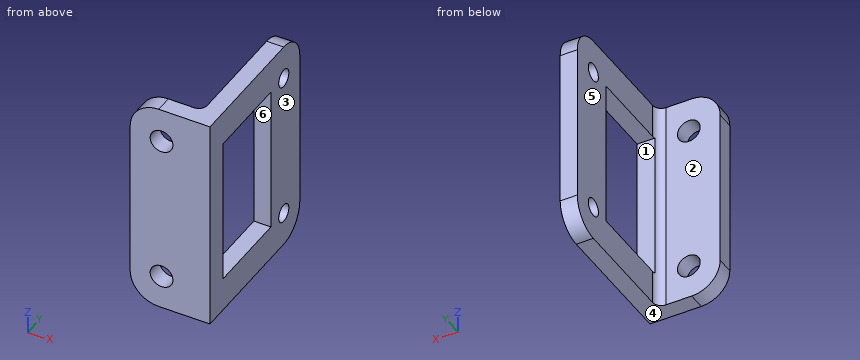
from build123d import *

# Parameters (mm, degrees)
BOSS_EXTRUDE1_DEPTH     = 19
CUT_EXTRUDE1_DEPTH      = 33.954514107
CUT_EXTRUDE1_DEPTH_BACK = 33.954514107
SKETCH2_R               = 2
SKETCH3_R               = 1.575
SKETCH3_W               = 26
SKETCH3_H               = 15
CUT_EXTRUDE2_DEPTH      = 36.580893749
FILLET1_R               = 1.5
FILLET2_R               = 5


with BuildPart() as part:
    # Sketch1 → Boss-Extrude1 (new, symmetric)
    with BuildSketch(Plane.XY):
        Polygon((0, 0), (4, 0), (4, 28), (1, 28), (1, 3), (-10, 3), (-10, 0), align=None)
    extrude(amount=BOSS_EXTRUDE1_DEPTH, both=True)

    # Sketch2 → Cut-Extrude1 (cut, two sides: drawn at the far end of the back side and taken through both)
    with BuildSketch(Plane(origin=(0, 3, 0), x_dir=(1, 0, 0), z_dir=(0, 1, 0)).offset(-CUT_EXTRUDE1_DEPTH_BACK)):
        with Locations(Location((-4.5, 13, 0), (0, 0, 180))):
            Circle(SKETCH2_R)
        with Locations((-4.5, -13)):
            Circle(SKETCH2_R)
    extrude(amount=CUT_EXTRUDE1_DEPTH + CUT_EXTRUDE1_DEPTH_BACK, mode=Mode.SUBTRACT)

    # Sketch3 → Cut-Extrude2 (cut, through all)
    with BuildSketch(Plane.ZY.offset(-1)):
        with Locations((-13, 23)):
            Circle(SKETCH3_R)
        with Locations(Location((13, 23, 0), (0, 0, 180))):
            Circle(SKETCH3_R)
        with Locations((0, 11.5)):
            Rectangle(SKETCH3_W, SKETCH3_H)
    extrude(amount=-CUT_EXTRUDE2_DEPTH, mode=Mode.SUBTRACT)

    # Fillet1
    # the kernel refuses this fillet: 1.5 mm, written as the material it adds along each edge
    with BuildSketch(Plane(origin=(1, 3, -19), x_dir=(0, 1, 0), z_dir=(0, 0, 1))) as fillet1_piece_1_section:
        with BuildLine():
            CenterArc((FILLET1_R, FILLET1_R), FILLET1_R, 180, 90)
            Line((0, FILLET1_R), (0, 0))
            Line((0, 0), (FILLET1_R, 0))
        make_face()
    fillet1_piece_1 = extrude(amount=38, mode=Mode.PRIVATE)
    fillet1_piece_1 = split(fillet1_piece_1, bisect_by=Plane(origin=(0.995303959, 4, -16), z_dir=(0, 1, 0)), keep=Keep.TOP, mode=Mode.PRIVATE)
    fillet1_piece_1 = split(fillet1_piece_1, bisect_by=Plane(origin=(0.995303959, 4.189014255, -13), z_dir=(0, 0, -1)), keep=Keep.TOP, mode=Mode.PRIVATE)
    add(fillet1_piece_1)
    with BuildSketch(Plane(origin=(1, 3, -19), x_dir=(0, 1, 0), z_dir=(0, 0, 1))) as fillet1_piece_2_section:
        with BuildLine():
            CenterArc((FILLET1_R, FILLET1_R), FILLET1_R, 180, 90)
            Line((0, FILLET1_R), (0, 0))
            Line((0, 0), (FILLET1_R, 0))
        make_face()
    fillet1_piece_2 = extrude(amount=38, mode=Mode.PRIVATE)
    fillet1_piece_2 = split(fillet1_piece_2, bisect_by=Plane(origin=(0.642494848, 4, -16), z_dir=(0, -1, 0)), keep=Keep.TOP, mode=Mode.PRIVATE)
    fillet1_piece_2 = split(fillet1_piece_2, bisect_by=Plane(origin=(0.642494848, 3.294160002, -13), z_dir=(0, 0, -1)), keep=Keep.TOP, mode=Mode.PRIVATE)
    add(fillet1_piece_2)
    with BuildSketch(Plane(origin=(1, 3, -19), x_dir=(0, 1, 0), z_dir=(0, 0, 1))) as fillet1_piece_3_section:
        with BuildLine():
            CenterArc((FILLET1_R, FILLET1_R), FILLET1_R, 180, 90)
            Line((0, FILLET1_R), (0, 0))
            Line((0, 0), (FILLET1_R, 0))
        make_face()
    fillet1_piece_3 = extrude(amount=38, mode=Mode.PRIVATE)
    fillet1_piece_3 = split(fillet1_piece_3, bisect_by=Plane(origin=(0.642494848, 4, 0), z_dir=(0, -1, 0)), keep=Keep.TOP, mode=Mode.PRIVATE)
    fillet1_piece_3 = split(fillet1_piece_3, bisect_by=Plane(origin=(0.642494848, 3.294160002, -13), z_dir=(0, 0, 1)), keep=Keep.TOP, mode=Mode.PRIVATE)
    fillet1_piece_3 = split(fillet1_piece_3, bisect_by=Plane(origin=(0.642494848, 3.294160002, 13), z_dir=(0, 0, -1)), keep=Keep.TOP, mode=Mode.PRIVATE)
    add(fillet1_piece_3)
    with BuildSketch(Plane(origin=(1, 3, -19), x_dir=(0, 1, 0), z_dir=(0, 0, 1))) as fillet1_piece_4_section:
        with BuildLine():
            CenterArc((FILLET1_R, FILLET1_R), FILLET1_R, 180, 90)
            Line((0, FILLET1_R), (0, 0))
            Line((0, 0), (FILLET1_R, 0))
        make_face()
    fillet1_piece_4 = extrude(amount=38, mode=Mode.PRIVATE)
    fillet1_piece_4 = split(fillet1_piece_4, bisect_by=Plane(origin=(0.995303959, 4, 16), z_dir=(0, 1, 0)), keep=Keep.TOP, mode=Mode.PRIVATE)
    fillet1_piece_4 = split(fillet1_piece_4, bisect_by=Plane(origin=(0.995303959, 4.189014255, 13), z_dir=(0, 0, 1)), keep=Keep.TOP, mode=Mode.PRIVATE)
    add(fillet1_piece_4)
    with BuildSketch(Plane(origin=(1, 3, -19), x_dir=(0, 1, 0), z_dir=(0, 0, 1))) as fillet1_piece_5_section:
        with BuildLine():
            CenterArc((FILLET1_R, FILLET1_R), FILLET1_R, 180, 90)
            Line((0, FILLET1_R), (0, 0))
            Line((0, 0), (FILLET1_R, 0))
        make_face()
    fillet1_piece_5 = extrude(amount=38, mode=Mode.PRIVATE)
    fillet1_piece_5 = split(fillet1_piece_5, bisect_by=Plane(origin=(0.642494848, 4, 16), z_dir=(0, -1, 0)), keep=Keep.TOP, mode=Mode.PRIVATE)
    fillet1_piece_5 = split(fillet1_piece_5, bisect_by=Plane(origin=(0.642494848, 3.294160002, 13), z_dir=(0, 0, 1)), keep=Keep.TOP, mode=Mode.PRIVATE)
    add(fillet1_piece_5)

    # Fillet2
    fillet2_edges = [part.edges().sort_by_distance(p)[0] for p in [
        (2.5, 28, 19),
        (-10, 1.5, 19),
        (-10, 1.5, -19),
        (2.5, 28, -19),
    ]]
    fillet(fillet2_edges, radius=FILLET2_R)


solid = part.part
Build history of the part. All positions in model axes, mm. Face numbers are marked on the shaded views. A direction names the side the tool comes from. Coordinates: 2 decimals unless noted, no trailing zeros. Write each loop counter-clockwise with the first axis right and the second up, starting at its lowest first coordinate (ties: lowest second). Pieces come first, ordered by that corner, then holes. Notation, with made-up numbers: (82, 56) -> (87, 56) arc R24 cw to (87, 81) -> close; hole circle Ø5 at (81, -36). An arc over 180 degrees is marked (long way). Use CSV: the item, a comma, the result in double quotes. Start each with the question number.
Q1. 3-axis set-ups, long thin cutter, end or side, ignore diameter. For the marked faces 1, 2 and 3: which of +Z, -Z, +X, -X, +Y, -Y reach the whole face in a straight line?
Q2. Cut at B-B, the plane x = -4.5. List the corners of the cut face in (y, z).
Q3. Pull direction Z, two halves, no side cores. Call the marked faces 4, 5 and 6: released by +Z, released by -Z, zero draft, split by the parting line, or undercut.
Q4. Cut at A-A, the plane y = 9.5. List the corners of the cut face in (x, z).
Q5. Drill centre lines: probe 1 along Z at (x, y) = (-4.5, 1.8); probe 2 along Z at (x, y) = (2.25, 4.25); probe 3 along X at (y, z) = (21, 9.5). Where is each one in solid material? Low to high.
Q6. Cut at C-C, the plane z = 0.5. List the corners of the cut face in (x, y).
Q7. Cut at D-D, the plane x = 1.75. List the corners of the cut face in (y, z) (3 decimals).
Q8. Flat gauge pins, fed straight in: pin 1 Ø2 at (x, z) = (-6.5, -7.5) entering from +Y; pin 2 Ø3.5 at (y, z) = (23, 13) entering from -X; pin 3 Ø3.5 at (x, z) = (-4.5, -13) entering from +Y. Where does each tip first touch, or does it go through?
Checked values:
1,face 1,"+X, -X"
1,face 2,"+Z, -Z, -X, +Y"
1,face 3,"+Z, -Z, +X, +Y, -Y"
2,outline,"(0, -19) -> (3, -19) -> (3, -15) -> (0, -15) -> close; (0, -11) -> (3, -11) -> (3, 11) -> (0, 11) -> close; (0, 15) -> (3, 15) -> (3, 19) -> (0, 19) -> close"
3,face 4,"released by -Z"
3,face 5,"zero draft"
3,face 6,"undercut"
4,outline,"(1, -19) -> (4, -19) -> (4, -13) -> (1, -13) -> close; (1, 13) -> (4, 13) -> (4, 19) -> (1, 19) -> close"
5,probe 1,"z = -19 to -15, -11 to 11, 15 to 19"
5,probe 2,"z = -19 to -13, 13 to 19"
5,probe 3,"x = 1 to 4"
6,outline,"(-10, 0) -> (4, 0) -> (4, 4) -> (0.91, 4) arc R1.5 cw to (-0.5, 3) -> (-10, 3) -> close; (1, 19) -> (4, 19) -> (4, 28) -> (1, 28) -> close"
7,outline,"(0, -19) -> (23, -19) arc R5 ccw to (28, -14) -> (28, 14) arc R5 ccw to (23, 19) -> (0, 19) -> close; hole (4, -13) -> (19, -13) -> (19, 13) -> (4, 13) -> close; hole circle Ø3.15 at (23, -13); hole circle Ø3.15 at (23, 13)"
8,pin 1,"stops at y = 3"
8,pin 2,"stops at x = 1"
8,pin 3,"passes through"
